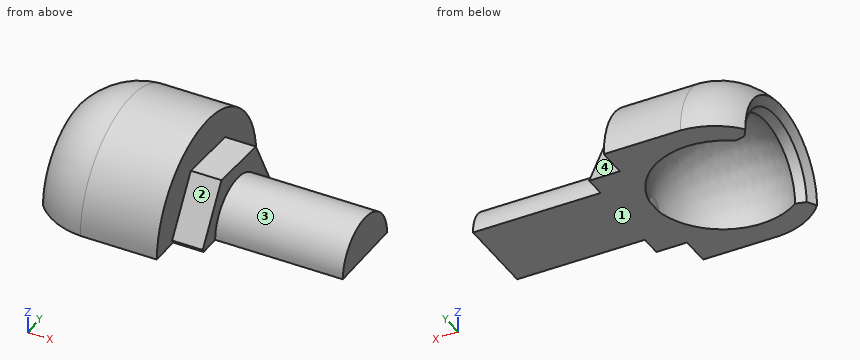
from build123d import *

# Parameters (mm, degrees)
Y_KSEKLIK_EKSTR_ZYON1_DEPTH = 6
IZIM3_R                     = 8
BOSS_EXTRUDE1_DEPTH         = 25
SKETCH3_W                   = 31.552756476
SKETCH3_H                   = 60.481987933
CUT_EXTRUDE2_DEPTH          = 67


with BuildPart() as part:
    # Çizim1 → Döndür1 (revolve)
    with BuildSketch(Plane.XY):
        with BuildLine():
            Line((-25, 13), (-23.9, 11.25))
            Line((-23.9, 11.25), (-21.913347284, 10.75))
            ThreePointArc((-21.913347284, 10.75), (-8.560110762, 12.229864882), (-0.153484939, 1.75))
            Line((-0.153484939, 1.75), (-0.153484939, 0))
            Line((-0.153484939, 0), (0, 0))
            Line((0, 0), (0, 18))
            Line((0, 18), (-15, 18))
            ThreePointArc((-15, 18), (-20.524257416, 16.548514832), (-25, 13))
        make_face()
    revolve(axis=Axis((-0.153484939, 0, 0), (1, 0, 0)))

    # Çizim2 → Yükseklik-Ekstrüzyon1 (add)
    with BuildSketch(Plane(origin=(0, 0, 0), x_dir=(0, 0, -1), z_dir=(1, 0, 0))):
        Polygon((-0.613358655, -12.484575463), (10.505280179, -6.773471909), (11.118638834, 5.711103554), (0.613358655, 12.484575463), (-10.505280179, 6.773471909), (-11.118638834, -5.711103554), align=None)
    extrude(amount=Y_KSEKLIK_EKSTR_ZYON1_DEPTH)

    # Çizim3 → Boss-Extrude1 (add)
    with BuildSketch(Plane(origin=(6, 0, 0), x_dir=(0, 0, -1), z_dir=(1, 0, 0))):
        Circle(IZIM3_R)
    extrude(amount=BOSS_EXTRUDE1_DEPTH)

    # Sketch3 → Cut-Extrude2 (cut)
    with BuildSketch(Plane(origin=(31, 0, 0), x_dir=(0, 0, -1), z_dir=(1, 0, 0))):
        with Locations((15.776378238, -7.418738571)):
            Rectangle(SKETCH3_W, SKETCH3_H)
    extrude(amount=-CUT_EXTRUDE2_DEPTH, mode=Mode.SUBTRACT)


solid = part.part
Can you work these out from the model? Positions are in its coordinate system, mm. Face numbers are marked on the shaded views. A direction names the side the tool comes from. Give positions to 0.01 mm unless a question says otherwise; leave off trailing zeros. Order: outer loops, then holes, each group sorted by start corner. A loop starts at its lowest first (then second) coordinate and runs counter-clockwise, first axis right, second up. Notation, with made-up numbers: (19.25, 69.5) - (60.25, 69.5) arc R6 ccw to (60.25, 75.5) - close; hole circle Ø11 at (-37.5, 81.5). An arc over 180 degrees is marked (long way). Write each question's results on one line, items separated by ' | '.
1) Please list where these lines run through material, in increasing order: line 1 along X through (y, z) = (4.5, 10.5); line 2 along Y through (x, z) = (27, 6.75); line 3 along Y through (x, z) = (-18, 13). Write a range as [from, to].
Final values:
line 1: x = [-24.01, -20.86], [-6.92, 6] | line 2: y = [-4.29, 4.29] | line 3: y = [-11.74, 11.74]
2) On a 3-axis mill with a long thin cutter (end or side, diameter ignored), from which of +Z, -Z, +X, -X, +Y, -Y can I reach the whole of each face in a straight line? I mean the marked faces 1, 2, 3 and 4. Say none if no direction works.
Final values:
face 1: -Z, +X, -X, +Y, -Y | face 2: +Z, +X, -Y | face 3: +Z, +X | face 4: +Z, +X, +Y
3) I'm going to push flat-ended pins straight in: pin 1 Ø1.5 at (x, y) = (-10.5, -6) entering from +Z; pin 2 Ø1.5 at (y, z) = (-10, 14.5) entering from -X; pin 3 Ø8 at (y, z) = (14, 12) entering from -X. Where does each tip first touch, or does it pass through?
Final values:
pin 1: stops at z = 17.22 | pin 2: stops at x = -19.85 | pin 3: stops at x = -23.62
4) Suppose I cut it at A-A, the plane x = 18. Write out the boundary of the cut face in (y, z), then the cut area to 3 significant figures.
Final values:
outline: (-8, 0) - (8, 0) arc R8 ccw to start | area: 101 mm^2
